Here's how the part is built. I have some questions about the finished solid (model axes, mm). A direction names the side the tool comes from. Give positions to 0.01 mm unless a question says otherwise; leave off trailing zeros. Loops run counter-clockwise (first coordinate to the right, second up) from the corner with the lowest first, then second, coordinate; pieces in that order, holes last. Notation, with made-up numbers: (51, 82.25) - (76, 82.25) arc R23 ccw to (76, 117.25) - close; hole circle Ø11 at (40, 84.25). An arc over 180 degrees is marked (long way). Return JSON: item names as keys, results as strings. Group by question number.
(1) For P1, Ø0.7, axis at x = -139, z = -143, coming from the -Y side; P2, Ø7.5, axis at x = 114.3, z = -203.2, coming from the -Y side; P3, Ø4, axis at y = -17.48, z = -23.83, coming from the +X side; P4, Ø8, axis at x = -68, y = -7.5, coming from the +Z side, each with a flat end and sliding along its axis, tell me the tip position at first contact or that it passes through.
(2) If we section it at B-B (y = -10.5): Please give me the cut outline in (x, z), then the cut area to 3 significant figures.
(3) On a 3-axis mill with a long thin cutter (end or side, diameter ignored), from which of +Z, -Z, +X, -X, +Y, -Y can I reach the whole of each face in a straight line? I mean faces 1 (the flat face through (2, 2, -227.025)), 2 (the flat face through (3, 0, -112)). Say none if no direction works.
(4) If we section it at D-D (z = -126.5): Please give me the cut outline in (x, y).
(5) If we section it at A-A (z = -76.2): Please give me the cut outline in (x, y) (3 decimals), then the cut area to 3 significant figures.
(6) I need wall thicknesses on probe 1 along X at (y, z) = (-5.5, -213.5); probe 2 along X at (y, z) = (1, -203); probe 3 along Z at (x, y) = (114, 1). Which ranges of each line are inside material? Lowest first, please. Write a range as [from, to].
(7) If we mould it in two halves opening along Y, with no side actions, what happens to faces 3 (the flat face through (-1, 2.286, -112)), 4 (the cylindrical face through (140.859, -17.336, -192.103)), 5 (the cylindrical face through (140.859, -17.336, -20.653)), 6 (the flat face through (1, 2, 0))? For each: released by +Y, released by -Y, zero draft, split by the parting line, or undercut.
(8) If we section it at C-C (x = 76.2): Please give me the cut outline in (y, z) (3 decimals), then the cut area to 3 significant figures.
```python
from build123d import *

# Parameters (mm, degrees)
BASE_FLANGE1_DEPTH = 227.0252
CUT_EXTRUDE1_REACH = 271.924
SKETCH2_R          = 28.575
SKETCH2_R_2        = 3.175
SKETCH3_R          = 3.175
CUT_EXTRUDE2_DEPTH = 7.62
FILLET1_R          = 0.762
CUT_EXTRUDE3_DEPTH = 270.923905809


# Sheet-metal steps are written as plain solids
with BuildPart() as part:
    # Sketch1 → Base-Flange1 (new body)
    with BuildSketch(Plane(origin=(0, 0, 0), x_dir=(-1, 0, 0), z_dir=(0, 0, -1))):
        with BuildLine():
            Line((-139.7, -31.75), (-139.7, -1.7272))
            ThreePointArc((-139.7, -1.7272), (-139.194114832, -0.505885168), (-137.9728, 0))
            Line((-137.9728, 0), (135.6868, 0))
            ThreePointArc((135.6868, 0), (136.908114832, -0.505885168), (137.414, -1.7272))
            Line((137.414, -1.7272), (137.414, -19.05))
            Line((137.414, -19.05), (139.7, -19.05))
            Line((139.7, -19.05), (139.7, -1.7272))
            ThreePointArc((139.7, -1.7272), (138.524560934, 1.110560934), (135.6868, 2.286))
            Line((135.6868, 2.286), (-137.9728, 2.286))
            ThreePointArc((-137.9728, 2.286), (-140.810560934, 1.110560934), (-141.986, -1.7272))
            Line((-141.986, -1.7272), (-141.986, -31.75))
            Line((-141.986, -31.75), (-139.7, -31.75))
        make_face()
    extrude(amount=BASE_FLANGE1_DEPTH)

    # Sketch2 → Cut-Extrude1 (cut, up to next)
    with BuildSketch(Plane(origin=(0, 2.286, 0), x_dir=(1, 0, 0), z_dir=(0, 1, 0)), mode=Mode.PRIVATE) as cut_extrude1_sk1:
        with Locations(Location((-76.2, 76.2, 0), (0, 0, 270))):
            Circle(SKETCH2_R)
    cut_extrude1_tool1 = extrude(cut_extrude1_sk1.sketch, amount=-CUT_EXTRUDE1_REACH, mode=Mode.PRIVATE) & part.part
    # Sketch2 → Cut-Extrude1 (cut, up to next)
    with BuildSketch(Plane(origin=(0, 2.286, 0), x_dir=(1, 0, 0), z_dir=(0, 1, 0)), mode=Mode.PRIVATE) as cut_extrude1_sk2:
        with Locations(Location((76.2, 76.2, 0), (0, 0, 270))):
            Circle(SKETCH2_R)
    cut_extrude1_tool2 = extrude(cut_extrude1_sk2.sketch, amount=-CUT_EXTRUDE1_REACH, mode=Mode.PRIVATE) & part.part
    # Sketch2 → Cut-Extrude1 (cut, up to next)
    with BuildSketch(Plane(origin=(0, 2.286, 0), x_dir=(1, 0, 0), z_dir=(0, 1, 0)), mode=Mode.PRIVATE) as cut_extrude1_sk3:
        with Locations(Location((114.3, 203.2, 0), (0, 0, 270))):
            Circle(SKETCH2_R_2)
    cut_extrude1_tool3 = extrude(cut_extrude1_sk3.sketch, amount=-CUT_EXTRUDE1_REACH, mode=Mode.PRIVATE) & part.part
    # Sketch2 → Cut-Extrude1 (cut, up to next)
    with BuildSketch(Plane(origin=(0, 2.286, 0), x_dir=(1, 0, 0), z_dir=(0, 1, 0)), mode=Mode.PRIVATE) as cut_extrude1_sk4:
        with Locations(Location((-114.3, 203.2, 0), (0, 0, 270))):
            Circle(SKETCH2_R_2)
    cut_extrude1_tool4 = extrude(cut_extrude1_sk4.sketch, amount=-CUT_EXTRUDE1_REACH, mode=Mode.PRIVATE) & part.part
    add(cut_extrude1_tool1.solids().sort_by_distance((-76.2, 2.286, -76.2))[0], mode=Mode.SUBTRACT)
    add(cut_extrude1_tool2.solids().sort_by_distance((76.2, 2.286, -76.2))[0], mode=Mode.SUBTRACT)
    add(cut_extrude1_tool3.solids().sort_by_distance((114.3, 2.286, -203.2))[0], mode=Mode.SUBTRACT)
    add(cut_extrude1_tool4.solids().sort_by_distance((-114.3, 2.286, -203.2))[0], mode=Mode.SUBTRACT)

    # Sketch3 → Cut-Extrude2 (cut)
    with BuildSketch(Plane(origin=(141.986, 0, 0), x_dir=(0, 0, -1), z_dir=(1, 0, 0))):
        with Locations((23.8252, -17.4752)):
            Circle(SKETCH3_R)
        with Locations((195.2752, -17.4752)):
            Circle(SKETCH3_R)
    extrude(amount=-CUT_EXTRUDE2_DEPTH, mode=Mode.SUBTRACT)

    # Fillet1
    fillet1_edges = [part.edges().sort_by_distance(p)[0] for p in [
        (140.843, -31.75, 0),
        (-138.557, -19.05, 0),
        (140.843, -31.75, -227.0252),
        (-138.557, -19.05, -227.0252),
    ]]
    fillet(fillet1_edges, radius=FILLET1_R)

    # Sketch4 → Cut-Extrude3 (cut, through all)
    with BuildSketch(Plane(origin=(0, 2.286, 0), x_dir=(1, 0, 0), z_dir=(0, 1, 0))):
        Polygon((150.619782866, 10.665476011), (128.807714722, -11.146592133), (150.619782866, -11.146592133), align=None)
    extrude(amount=-CUT_EXTRUDE3_DEPTH, mode=Mode.SUBTRACT)


solid = part.part
```
Values:
{
 "1": {"P1": "y = -19.05", "P2": "y = 0", "P3": "x = -137.41", "P4": "through"},
 "2": {"outline": "(-139.7, -227.03) - (-137.41, -227.03) - (-137.41, 0) - (-139.7, 0) - close; (139.7, -227.03) - (141.99, -227.03) - (141.99, -2.03) - (139.95, 0) - (139.7, 0) - close", "area": "1,040 mm2"},
 "3": {"face 1": "-Z, +X, -X, +Y, -Y", "face 2": "+Z, -Z, -Y"},
 "4": {"outline": "(-139.7, -19.05) - (-137.41, -19.05) - (-137.41, -1.73) arc R1.73 cw to (-135.69, 0) - (137.97, 0) arc R1.73 cw to (139.7, -1.73) - (139.7, -31.75) - (141.99, -31.75) - (141.99, -1.73) arc R4.01 ccw to (137.97, 2.29) - (-135.69, 2.29) arc R4.01 ccw to (-139.7, -1.73) - close"},
 "5": {"outline": "(-139.7, -19.05) - (-137.414, -19.05) - (-137.414, -1.727) arc R1.727 cw to (-135.687, 0) - (-104.775, 0) - (-104.775, 2.286) - (-135.687, 2.286) arc R4.013 ccw to (-139.7, -1.727) - close; (-47.625, 0) - (47.625, 0) - (47.625, 2.286) - (-47.625, 2.286) - close; (104.775, 0) - (137.973, 0) arc R1.727 cw to (139.7, -1.727) - (139.7, -31.75) - (141.986, -31.75) - (141.986, -1.727) arc R4.013 ccw to (137.973, 2.286) - (104.775, 2.286) - close", "area": "493 mm2"},
 "6": {"probe 1": "[-139.7, -137.41], [139.7, 141.99]", "probe 2": "[-138.63, -117.47], [-111.13, 111.13], [117.47, 140.92]", "probe 3": "[-227.03, -206.36], [-200.04, 0]"},
 "7": {"face 3": "released by +Y", "face 4": "undercut", "face 5": "undercut", "face 6": "zero draft"},
 "8": {"outline": "(0, -227.025) - (2.286, -227.025) - (2.286, -104.775) - (0, -104.775) - close; (0, -47.625) - (2.286, -47.625) - (2.286, 0) - (0, 0) - close", "area": "388 mm2"}
}
